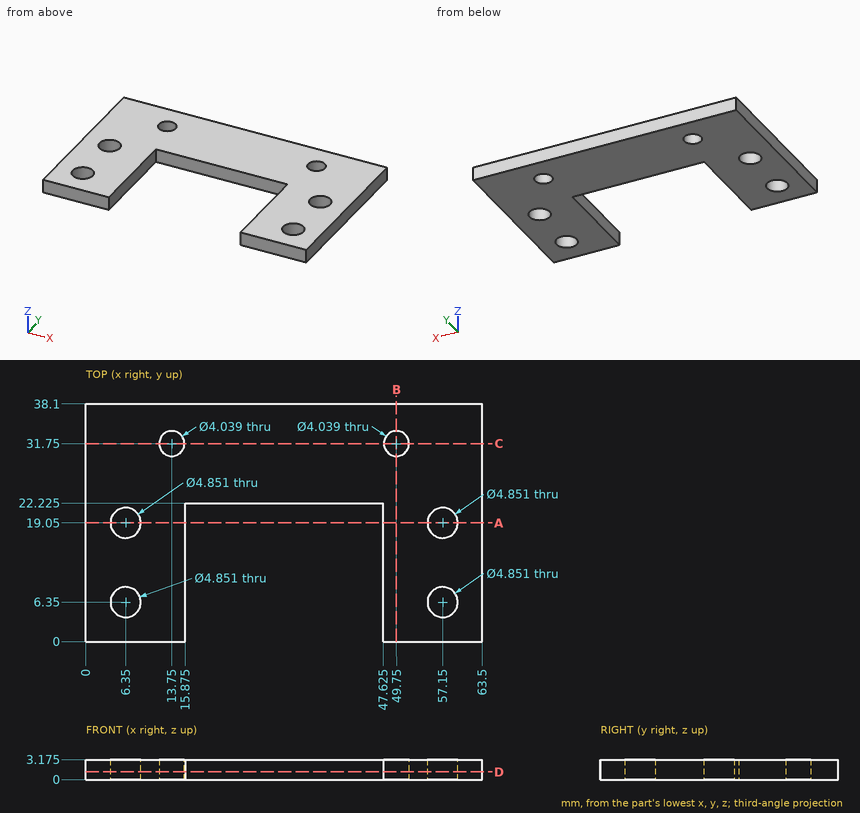
Here's the drawing with two shaded views (mm, measured from the low corner). I have some questions. Give positions to 0.01 mm unless a question says otherwise; leave off trailing zeros. Loops run counter-clockwise (first coordinate to the right, second up) from the corner with the lowest first, then second, coordinate; pieces in that order, holes last. Notation, with made-up numbers: M -26.5,-5.75 L 12.5,-5.75 A24 ccw 12.5,30.25 Z; hole C 32,17 d2. An arc over 180 degrees is marked long. Use one line per item in the form item = value. Start each with the question number.
(1) I want a section at C-C, the plane y = 31.75. Write out the boundary of the cut face in (x, z) (1 decimal), and give its area (3 significant figures).
(2) I want a section at D-D, the plane z = 1.25. State how many separate pieces and enclosed holes the cut face has, and give its area (3 significant figures).
(3) I'm going to push flat-ended pins straight in: P1, Ø1.6, axis at x = 34, z = 1, coming from the -Y side (3 decimals); P2, Ø4, axis at x = 57.15, y = 6.35, coming from the -Z side. Where does each tip first touch, or does it pass through?
(4) Please list where these lines run through material, in increasing order: line 1 (Y direction, x = 6.35, z = 1.25) (1 decimal); line 2 (X direction, y = 19, z = 1.4) (1 decimal); line 3 (X direction, y = 18.5, z = 0.65) (1 decimal).
(5) I want a section at A-A, the plane y = 19.05. Write out the boundary of the cut face in (x, z) (1 decimal).
(6) I want a section at B-B, the plane x = 49.75. Write out the boundary of the cut face in (y, z) (1 decimal).
Worked out:
q1.outline = M 0,0 L 11.7,0 L 11.7,3.2 L 0,3.2 Z; M 15.8,0 L 47.7,0 L 47.7,3.2 L 15.8,3.2 Z; M 51.8,0 L 63.5,0 L 63.5,3.2 L 51.8,3.2 Z
q1.area = 176 mm²
q2.separate_pieces = 1
q2.enclosed_holes = 6
q2.area = 1,610 mm²
q3.P1 = 22.225
q3.P2 = through
q4.line_1 = 0 to 3.9, 8.8 to 16.6, 21.5 to 38.1
q4.line_2 = 0 to 3.9, 8.8 to 15.9, 47.6 to 54.7, 59.6 to 63.5
q4.line_3 = 0 to 4, 8.7 to 15.9, 47.6 to 54.8, 59.5 to 63.5
q5.outline = M 0,0 L 3.9,0 L 3.9,3.2 L 0,3.2 Z; M 8.8,0 L 15.9,0 L 15.9,3.2 L 8.8,3.2 Z; M 47.6,0 L 54.7,0 L 54.7,3.2 L 47.6,3.2 Z; M 59.6,0 L 63.5,0 L 63.5,3.2 L 59.6,3.2 Z
q6.outline = M 0,0 L 29.7,0 L 29.7,3.2 L 0,3.2 Z; M 33.8,0 L 38.1,0 L 38.1,3.2 L 33.8,3.2 Z
